Can you work these out from the model? Positions are in its coordinate system, mm. A direction names the side the tool comes from. Round coordinates to 2 decimals unless told otherwise and drop trailing zeros. Loops run counter-clockwise (first coordinate to the right, second up) from the corner with the lowest first, then second, coordinate; pieces in that order, holes last.
```python
from build123d import *

# Parameters (mm, degrees)
BOSS_EXTRU_1_DEPTH           = 30
ENL_V_MAT_EXTRU_1_DEPTH      = 354.730123116
ENL_V_MAT_EXTRU_1_DEPTH_BACK = 354.730123116
ESQUISSE2_R                  = 13
ESQUISSE3_W                  = 410
ESQUISSE3_H                  = 290
BOSS_EXTRU_2_DEPTH           = 230
CONG_1_R                     = 50


with BuildPart() as part:
    # Esquisse1 → Boss.-Extru.1 (new body)
    with BuildSketch(Plane.XY):
        Polygon((300, 185), (-300, 185), (-300, 145), (-205, 145), (-205, -145), (-300, -145), (-300, -185), (300, -185), (300, -145), (205, -145), (205, 145), (300, 145), align=None)
    extrude(amount=BOSS_EXTRU_1_DEPTH)

    # Esquisse2 → Enlèv. mat.-Extru.1 (cut, two sides: drawn at the far end of the back side and taken through both)
    with BuildSketch(Plane.XY.offset(30).offset(-ENL_V_MAT_EXTRU_1_DEPTH_BACK)):
        with Locations((-277.5, 165)):
            Circle(ESQUISSE2_R)
        with Locations((277.5, 165)):
            Circle(ESQUISSE2_R)
        with Locations((277.5, -165)):
            Circle(ESQUISSE2_R)
        with Locations((-277.5, -165)):
            Circle(ESQUISSE2_R)
    extrude(amount=ENL_V_MAT_EXTRU_1_DEPTH + ENL_V_MAT_EXTRU_1_DEPTH_BACK, mode=Mode.SUBTRACT)

    # Esquisse3 → Boss.-Extru.2 (add)
    with BuildSketch(Plane.XY.offset(30)):
        Rectangle(ESQUISSE3_W, ESQUISSE3_H)
    extrude(amount=BOSS_EXTRU_2_DEPTH)

    # Congé1
    cong_1_edges = [part.edges().sort_by_distance(p)[0] for p in [
        (-205, 0, 260),
        (205, 0, 260),
    ]]
    fillet(cong_1_edges, radius=CONG_1_R)


solid = part.part
```
(1) Suppose I cut it at A-A (y = 165). Write out the boundary of the cut face in (x, z).
(2) If I drill on line 1 (Y direction, x = 277.5, z = 12.5); line 2 (X direction, y = -165, z = 20.5); line 3 (X direction, y = -41.5, z = 199), over which ranges is the centre line in solid material (lowest first)?
(3) For pin 1 (15.5 mm diameter, centred on x = -277.5, y = 165, fed in from +Z) (3 decimals); pin 2 (5 mm diameter, centred on y = -107.5, z = 174.5, fed in from +X); pin 3 (10 mm diameter, centred on x = 88, z = 154, fed in from +Y); pin 4 (12 mm diameter, centred on x = -128.5, y = 163, fed in from +Z), each with a flat end and sliding along its axis, tell me the tip position at first contact or that it passes through.
(4) Suppose I cut it at D-D (z = 130.5). Write out the boundary of the cut face in (x, y).
(5) Suppose I cut it at B-B (x = -277.5). Write out the boundary of the cut face in (y, z), then the cut area to 3 significant figures.
(6) Which directions (+Z, -Z, +X, -X, +Y, -Y) give clear straight access to the entire face, cutting with the end or side of a thin tool? Please do faces 1 (the flat face through (-252, -145, 15)), 2 (the flat face through (-3, -145, 143)), 3 (the flat face through (-300, 165, 15)).
(7) We'd pull the mould along Y, two halves only. Please class faces 4 (the flat face through (4, 185, 15)), 5 (the flat face through (-4, -165, 30)), 6 (the cylindrical face through (267.184, 157.09, 14.79)): released by +Y, released by -Y, zero draft, split by the parting line, or undercut.
(8) Suppose I cut it at C-C (x = 132). Write out the boundary of the cut face in (y, z), then the cut area to 3 significant figures.
Check result:
1. outline: (-300, 0) - (-290.5, 0) - (-290.5, 30) - (-300, 30) - close; (-264.5, 0) - (264.5, 0) - (264.5, 30) - (-264.5, 30) - close; (290.5, 0) - (300, 0) - (300, 30) - (290.5, 30) - close
2. line 1: y = -185 to -178, -152 to -145, 145 to 152, 178 to 185
2. line 2: x = -300 to -290.5, -264.5 to 264.5, 290.5 to 300
2. line 3: x = -205 to 205
3. pin 1: passes through
3. pin 2: stops at x = 205
3. pin 3: stops at y = 145
3. pin 4: stops at z = 30
4. outline: (-205, -145) - (205, -145) - (205, 145) - (-205, 145) - close
5. outline: (-185, 0) - (-178, 0) - (-178, 30) - (-185, 30) - close; (-152, 0) - (-145, 0) - (-145, 30) - (-152, 30) - close; (145, 0) - (152, 0) - (152, 30) - (145, 30) - close; (178, 0) - (185, 0) - (185, 30) - (178, 30) - close
5. area: 840 mm2
6. face 1: +Z, -Z, -X
6. face 2: +Z, +X, -X, -Y
6. face 3: +Z, -Z, -X, +Y, -Y
7. face 4: released by +Y
7. face 5: zero draft
7. face 6: undercut
8. outline: (-185, 0) - (185, 0) - (185, 30) - (145, 30) - (145, 260) - (-145, 260) - (-145, 30) - (-185, 30) - close
8. area: 77,800 mm2
